from build123d import *

# Parameters (mm, degrees)
F1_DEPTH = 14.478
F2_R     = 6.629323
F2_R_2   = 5.937499
F4_DEPTH = 25.4
F5_DEPTH = 25.4
F6_DEPTH = 3.048
F7_R     = 3.492039
F8_DEPTH = 25.4


with BuildPart() as f1:
    # F0 (on Top) → F1 (new body)
    with BuildSketch(Plane.XY):
        Polygon((10.796952, 19.020916), (-12.118302, 18.542465), (-27.716025, 10.007861), (-27.716025, -23.280972), (27.209018, -23.280972), (27.209018, 12.181873), align=None)
    extrude(amount=F1_DEPTH)

    # F2 (on face) → F4 (cut)
    with BuildSketch(Plane.XY.offset(14.478)):
        with Locations((-12.274181, 2.999703)):
            Circle(F2_R)
        with Locations((13.71629, 0)):
            Circle(F2_R_2)
    extrude(amount=-F4_DEPTH, mode=Mode.SUBTRACT)

    # F3 (on face) → F5 (cut)
    with BuildSketch(Plane.XY.offset(14.478)):
        Polygon((-11.141166, -15.069095), (-19.911459, -8.22922), (-25.51602, -11.649158), (-12.556246, -21.756373), (13.60538, -21.756373), (24.986776, -14.877899), (21.591935, -9.078152), (12.803014, -15.069095), align=None)
        Polygon((20.893362, 7.999514), (21.07358, 11.019492), (10.318228, 14.986938), (9.316061, 12.270162), align=None)
        Polygon((-5.16953, 14.986938), (-18.105717, 12.270162), (-17.412947, 8.971472), (-4.192307, 11.747987), align=None)
    extrude(amount=-F5_DEPTH, mode=Mode.SUBTRACT)

    # F0 (on Top) → F6 (join)
    with BuildSketch(Plane.XY):
        Polygon((0, 30.222755), (-12.118302, 18.542465), (10.796952, 19.020916), align=None)
    extrude(amount=F6_DEPTH)

    # F7 (on face) → F8 (cut)
    with BuildSketch(Plane.XY.offset(3.048)):
        with Locations((-0.660675, 24.38261)):
            Circle(F7_R)
    extrude(amount=-F8_DEPTH, mode=Mode.SUBTRACT)


solid = f1.part
Read the model definition and answer for the solid it produces. Units are mm, in the model's axes. A direction names the side the tool comes from. Round coordinates to 2 decimals unless told otherwise and drop trailing zeros. Order: outer loops, then holes, each group sorted by start corner. A loop starts at its lowest first (then second) coordinate and runs counter-clockwise, first axis right, second up.
1) The mould has two halves that part along Y. Classify faces 3 (the face through (15.024, 10.165, 7.34)), 4 (the face through (19.118, 15.554, 7.138)), 5 (the face through (-1.6, 20.5, 3.048)): released by +Y, released by -Y, zero draft, split by the parting line, or undercut.
2) The part is cut by section A-A on x = 16.5. Write down the section's boundary in (y, z), plus the area to 3 significant figures.
3) For faces 1 (the face through (-15.46, -11.7, 7.34)), 2 (the face through (-5.974, 24.464, 1.503)), determine the directions among +Z, -Z, +X, -X, +Y, -Y from which every point of the face is accessible in a straight line to the end or side of a thin tool.
4) The part is cut by section B-B on y = -16. Write down the section's boundary in (x, z).
5) Flat-ended cylindrical pins translate along their axes: pin 1 (9 mm diameter, centred on x = -0.66, y = 24.38, fed in from -Z); pin 2 (1.5 mm diameter, centred on x = 2, z = 6, fed in from +Y); pin 3 (5 mm diameter, centred on x = 18.5, z = 8, fed in from +Y); pin 4 (12 mm diameter, centred on x = -12.27, y = 3, fed in from -Z). Find the tip coordinate at first contact, or state that the pin passes through.
6) Straight lines are drawn through the part: L1, parallel to X at y = -13, z = 13.5; L2, parallel to Y at x = 12.5, z = 5.5; L3, parallel to Y at x = 18.5, z = 11.25. For each, find the intervals that lie inside material, in ascending order.
7) The part is cut by section C-C on z = 1.5. Write down the section's boundary in (x, y) (1 decimal), plus the area to 3 significant figures.
8) The part is cut by section D-D on x = -22.5. Write down the section's boundary in (y, z).
Resolved:
1. face 3: undercut
1. face 4: released by +Y
1. face 5: zero draft
2. outline: (-23.28, 0) - (-20.01, 0) - (-20.01, 14.48) - (-23.28, 14.48) - close; (-12.55, 0) - (-5.24, 0) - (-5.24, 14.48) - (-12.55, 14.48) - close; (5.24, 0) - (9.62, 0) - (9.62, 14.48) - (5.24, 14.48) - close; (12.71, 0) - (16.64, 0) - (16.64, 14.48) - (12.71, 14.48) - close
2. area: 274 mm2
3. face 1: +Z, -Z
3. face 2: +Z, -Z, -X, +Y
4. outline: (-27.72, 0) - (-19.94, 0) - (-19.94, 14.48) - (-27.72, 14.48) - close; (23.13, 0) - (27.21, 0) - (27.21, 14.48) - (23.13, 14.48) - close
5. pin 1: stops at z = 0
5. pin 2: stops at y = 18.85
5. pin 3: stops at y = 16.85
5. pin 4: passes through
6. L1: x = -27.72 to -23.78, -13.79 to 15.84, 23.89 to 27.21
6. L2: y = -23.28 to -21.76, -15.07 to -5.81, 5.81 to 11.1, 14.18 to 18.31
6. L3: y = -23.28 to -18.8, -11.19 to -3.52, 3.52 to 8.88, 11.97 to 15.81
7. outline: (-27.7, -23.3) - (27.2, -23.3) - (27.2, 12.2) - (10.8, 19) - (0, 30.2) - (-12.1, 18.5) - (-27.7, 10) - close; hole (-25.5, -11.6) - (-12.6, -21.8) - (13.6, -21.8) - (25, -14.9) - (21.6, -9.1) - (12.8, -15.1) - (-11.1, -15.1) - (-19.9, -8.2) - close; hole circle Ø13.3 at (-12.3, 3); hole (-18.1, 12.3) - (-17.4, 9) - (-4.2, 11.7) - (-5.2, 15) - close; hole circle Ø7 at (-0.7, 24.4); hole circle Ø11.9 at (13.7, 0); hole (9.3, 12.3) - (20.9, 8) - (21.1, 11) - (10.3, 15) - close
7. area: 1,620 mm2
8. outline: (-23.28, 0) - (-14, 0) - (-14, 14.48) - (-23.28, 14.48) - close; (-9.81, 0) - (12.86, 0) - (12.86, 14.48) - (-9.81, 14.48) - close
